from build123d import *

# Parameters (mm, degrees)
SKETCH1_W            = 35.169359311
SKETCH1_H            = 6
BOSS_EXTRUDE1_DEPTH  = 25
SKETCH2_W            = 35.169359311
SKETCH2_H            = 6
BOSS_EXTRUDE2_DEPTH  = 1.5
SKETCH3_W            = 35.169359311
SKETCH3_H            = 6
BOSS_EXTRUDE3_DEPTH  = 1.5
SKETCH4_W            = 41.262531498
SKETCH4_H            = 46.473158343
BOSS_EXTRUDE4_DEPTH  = 1.5
BOSS_EXTRUDE5_DEPTH  = 2
BOSS_EXTRUDE6_DEPTH  = 2
SKETCH8_W            = 9.078602689
SKETCH8_H            = 1
BOSS_EXTRUDE7_DEPTH  = 0.5
SKETCH9_W            = 9.078602689
SKETCH9_H            = 1
BOSS_EXTRUDE8_DEPTH  = 0.5
BOSS_EXTRUDE9_DEPTH  = 1.5
BOSS_EXTRUDE10_DEPTH = 1.5
SKETCH13_R           = 1.114440401
CUT_EXTRUDE1_DEPTH   = 10


with BuildPart() as part:
    # Sketch1 → Boss-Extrude1 (new body)
    with BuildSketch(Plane(origin=(0, 0, 0), x_dir=(0, 0, -1), z_dir=(1, 0, 0))):
        Polygon((-55.278617962, 72.850669778), (-46.200015273, 72.850669778), (-46.200015273, 78.4511375), (-55.278617962, 74.184840555), align=None)
        with Locations((-51.170377926, 69.850669778)):
            Rectangle(SKETCH1_W, SKETCH1_H)
        Polygon((-43.112055174, 72.850669778), (-33.58569827, 72.850669778), (-33.58569827, 73.967743314), (-43.112055174, 78.444452863), align=None)
    extrude(amount=BOSS_EXTRUDE1_DEPTH)

    # Sketch2 → Boss-Extrude2 (add)
    with BuildSketch(Plane(origin=(25, 0, 0), x_dir=(0, 0, -1), z_dir=(1, 0, 0))):
        with Locations((-51.170377926, 69.850669778)):
            Rectangle(SKETCH2_W, SKETCH2_H)
    extrude(amount=BOSS_EXTRUDE2_DEPTH)

    # Sketch3 → Boss-Extrude3 (add)
    with BuildSketch(Plane.ZY):
        with Locations((51.170377926, 69.850669778)):
            Rectangle(SKETCH3_W, SKETCH3_H)
    extrude(amount=BOSS_EXTRUDE3_DEPTH)

    # Sketch4 → Boss-Extrude4 (add)
    with BuildSketch(Plane.XZ.offset(-66.850669778)):
        with Locations((12.174758659, 50.720136909)):
            Rectangle(SKETCH4_W, SKETCH4_H)
    extrude(amount=BOSS_EXTRUDE4_DEPTH)

    # Sketch6 → Boss-Extrude5 (add)
    with BuildSketch(Plane(origin=(25, 0, 0), x_dir=(0, 0, -1), z_dir=(1, 0, 0))):
        Polygon((-55.278617962, 72.850669778), (-55.278617962, 74.184840555), (-46.200015273, 78.4511375), (-46.200015273, 72.850669778), align=None)
    extrude(amount=BOSS_EXTRUDE5_DEPTH)

    # Sketch7 → Boss-Extrude6 (add)
    with BuildSketch(Plane.ZY):
        Polygon((46.200015273, 72.850669778), (55.278617962, 72.850669778), (55.278617962, 74.184840555), (46.200015273, 78.4511375), align=None)
    extrude(amount=BOSS_EXTRUDE6_DEPTH)

    # Sketch8 → Boss-Extrude7 (add)
    with BuildSketch(Plane(origin=(26.5, 0, 0), x_dir=(0, 0, -1), z_dir=(1, 0, 0))):
        with Locations((-50.739316618, 72.350669778)):
            Rectangle(SKETCH8_W, SKETCH8_H)
    extrude(amount=BOSS_EXTRUDE7_DEPTH)

    # Sketch9 → Boss-Extrude8 (add)
    with BuildSketch(Plane.ZY.offset(1.5)):
        with Locations((50.739316618, 72.350669778)):
            Rectangle(SKETCH9_W, SKETCH9_H)
    extrude(amount=BOSS_EXTRUDE8_DEPTH)

    # Sketch10 → Boss-Extrude9 (add)
    with BuildSketch(Plane(origin=(25, 0, 0), x_dir=(0, 0, -1), z_dir=(1, 0, 0))):
        Polygon((-43.112055174, 72.850669778), (-33.58569827, 72.850669778), (-33.58569827, 73.967743314), (-43.112055174, 78.444452863), align=None)
    extrude(amount=BOSS_EXTRUDE9_DEPTH)

    # Sketch11 → Boss-Extrude10 (add)
    with BuildSketch(Plane.ZY):
        Polygon((33.58569827, 72.850669778), (43.112055174, 72.850669778), (43.112055174, 78.444452863), (33.58569827, 73.967743314), align=None)
    extrude(amount=BOSS_EXTRUDE10_DEPTH)

    # Sketch13 → Cut-Extrude1 (cut)
    with BuildSketch(Plane.XY.offset(55.278617962)):
        with Locations((12.5, 74.184840555)):
            Circle(SKETCH13_R)
    extrude(amount=-CUT_EXTRUDE1_DEPTH, mode=Mode.SUBTRACT)


solid = part.part
Part model, mm, in its own coordinate system. A direction names the side the tool comes from. Give positions to 0.01 mm unless a question says otherwise; leave off trailing zeros. Order: outer loops, then holes, each group sorted by start corner. A loop starts at its lowest first (then second) coordinate and runs counter-clockwise, first axis right, second up. Notation, with made-up numbers: (18, 45) - (23, 45) arc R10 cw to (23, 54) - close; hole circle Ø6 at (-27, -21). An arc over 180 degrees is marked (long way). One line per question, with ' | ' between items.
1. Band-saw the part on B-B on y = 74.75. List the corners of the cut face in (x, z), then the cut area to 3 significant figures.
Filled in:
outline: (-2, 46.2) - (11.54, 46.2) - (11.54, 54.08) - (-2, 54.08) - close; (-1.5, 35.25) - (26.5, 35.25) - (26.5, 43.11) - (-1.5, 43.11) - close; (13.46, 46.2) - (27, 46.2) - (27, 54.08) - (13.46, 54.08) - close | area: 433 mm²
2. Band-saw the part on A-A on x = 12.5. List the corners of the cut face in (y, z), then the cut area to 3 significant figures.
Filled in:
outline: (65.35, 27.48) - (66.85, 27.48) - (66.85, 33.59) - (73.97, 33.59) - (78.44, 43.11) - (72.85, 43.11) - (72.85, 46.2) - (73.07, 46.2) - (73.07, 55.28) - (72.85, 55.28) - (72.85, 68.76) - (66.85, 68.76) - (66.85, 73.96) - (65.35, 73.96) - close; (75.3, 46.2) - (78.45, 46.2) - (75.3, 52.91) - close | area: 325 mm²
3. Band-saw the part on D-D on x = 2.5. List the corners of the cut face in (y, z).
Filled in:
outline: (65.35, 27.48) - (66.85, 27.48) - (66.85, 33.59) - (73.97, 33.59) - (78.44, 43.11) - (72.85, 43.11) - (72.85, 46.2) - (78.45, 46.2) - (74.18, 55.28) - (72.85, 55.28) - (72.85, 68.76) - (66.85, 68.76) - (66.85, 73.96) - (65.35, 73.96) - close
4. Drop flat-ended pins along their axis: P1, Ø8, axis at x = -2, z = 38.5, coming from the +Y side; P2, Ø6, axis at y = 73.5, z = 48, coming from the -X side; P3, Ø5.5, axis at x = 10.5, y = 76.5, coming from the -Z side. Give the stop position or say it passes through.
Filled in:
P1: y = 78.14 | P2: x = -2 | P3: z = 33.59
5. Which spindle directions (+Z, -Z, +X, -X, +Y, -Y) get a long thin tool onto all of the face, cutting with end or side? Do faces 4 (the face through (27, 74, 50)), 5 (the face through (13, 76, 43.112)), 6 (the face through (13, 72.851, 62)). Say none if no direction does.
Filled in:
face 4: +Z, -Z, +X, +Y | face 5: +X, -X, +Y | face 6: +Z, +X, -X, +Y
6. Band-saw the part on C-C on z = 44. List the corners of the cut face in (x, y).
Filled in:
outline: (-8.46, 65.35) - (32.81, 65.35) - (32.81, 66.85) - (26.5, 66.85) - (26.5, 72.85) - (-1.5, 72.85) - (-1.5, 66.85) - (-8.46, 66.85) - close
7. Pull direction Z, two halves, no side cores. Call faces 1 (the face through (12.7, 76.24, 38.42)), 2 (the face through (13, 72.851, 45)), 3 (the face through (12, 65.351, 51)): +Z half, -Z half, draft (parallel to the pull), parting line (faces both ways), or undercut.
Filled in:
face 1: -Z half | face 2: undercut | face 3: draft
8. Drill centre lines: probe 1 along Z at (x, y) = (19, 73.75); probe 2 along X at (y, z) = (68, 48); probe 3 along Y at (x, z) = (2.5, 68.5). Where is each one in solid material? Low to high.
Filled in:
probe 1: 33.59 to 43.11, 46.2 to 55.28 | probe 2: -1.5 to 26.5 | probe 3: 65.35 to 72.85
